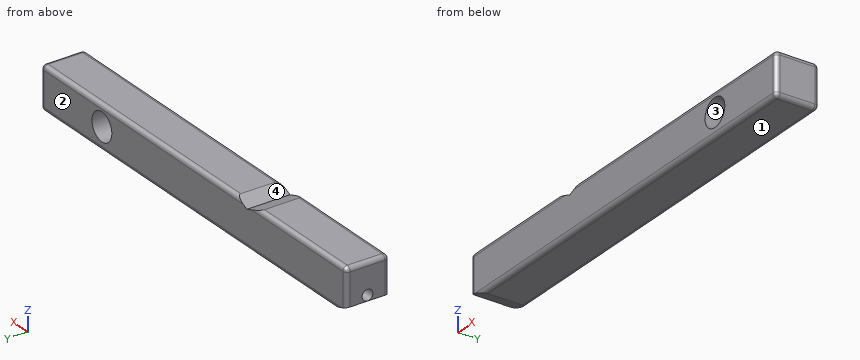
```python
from build123d import *

# Parameters (mm, degrees)
F0_R     = 3.25
F1_DEPTH = 10
F2_R     = 1.25
F3_DEPTH = 25
F4_R     = 1
F5_R     = 1


with BuildPart() as f1:
    # F0 (on Front) → F1 (new body)
    with BuildSketch(Plane.XZ):
        Polygon((-40.604423, 16.252205), (-36.365006, 14.785099), (59.395577, 14.785099), (59.395577, 24.785099), (-4.71925, 24.785099), (-8.140423, 23.253271), (-12.521202, 24.785099), (-40.604423, 24.785099), align=None)
        with Locations((39.395577, 20.006654)):
            Circle(F0_R, mode=Mode.SUBTRACT)
    extrude(amount=F1_DEPTH)

    # F2 (on face) → F3 (cut)
    with BuildSketch(Plane(origin=(-40.604423, 0, 0), x_dir=(0, -1, 0), z_dir=(-1, 0, 0))):
        with Locations((5, 17.535099)):
            Circle(F2_R)
    extrude(amount=-F3_DEPTH, mode=Mode.SUBTRACT)

    # F4
    f4_edges = [f1.edges().sort_by_distance(p)[0] for p in [
        (-26.562812, -10, 24.785099),
        (27.338164, -10, 24.785099),
        (27.338164, 0, 24.785099),
        (-26.562812, 0, 24.785099),
        (-40.604423, 0, 20.518652),
        (-40.604423, -5, 24.785099),
        (-40.604423, -10, 20.518652),
    ]]
    fillet(f4_edges, radius=F4_R)

    # F5
    f5_edges = [f1.edges().sort_by_distance(p)[0] for p in [
        (11.515286, -10, 14.785099),
        (11.515286, 0, 14.785099),
        (59.395577, -5, 24.785099),
        (59.395577, -0.292893, 24.492206),
        (59.395577, -9.707107, 24.492206),
        (59.395577, 0, 19.285099),
        (59.395577, -10, 19.285099),
        (59.395577, -5, 14.785099),
    ]]
    fillet(f5_edges, radius=F5_R)


solid = f1.part
```
Can you work these out from the model? Positions are in its coordinate system, mm. Face numbers are marked on the shaded views. Coordinates: 2 decimals unless noted, no trailing zeros. Loops run counter-clockwise (first coordinate to the right, second up) from the corner with the lowest first, then second, coordinate; pieces in that order, holes last. Notation, with made-up numbers: (-13, 18) - (32, 18) arc R10 ccw to (32, 36) - close; hole circle Ø10 at (-22, 23.5). An arc over 180 degrees is marked (long way). Answer as CSV lines item,"result". Start each with the question number.
1) Suppose I cut it at A-A (z = 22.25). Please give me the cut outline in (x, y), plus the area to 3 significant figures.
2) Suppose I cut it at C-C (x = -19). Please give me the cut outline in (y, z), plus the area to 3 significant figures.
3) Suppose I cut it at B-B (y = -5). Please give me the cut outline in (x, z) (3 decimals), plus the area to 3 significant figures.
4) Thinking about a two-plate mould opening in Z: for the marked faces 1, 2, 3 and 4, which applies, pulls with the +Z half, pulls with the -Z half, needs draft (parallel to the pull), parting line crosses it, or undercut?
5) For pin 1 (1.5 mm diameter, centred on y = -5, z = 17.54, fed in from -X), with a flat end and sliding along its axis, tell me the tip position at first contact or that it passes through.
6) I need wall thicknesses on line 1 (Z direction, x = -28.25, y = -5); line 2 (X direction, y = -8.25, z = 17.5); line 3 (X direction, y = -5, z = 22). Which ranges of each line are inside material? Lowest first, please. Write a range as from..to.
Check result:
1,outline,"(-40.6, -9) arc R1 ccw to (-39.6, -10) - (37.04, -10) - (37.04, 0) - (-39.6, 0) arc R1 ccw to (-40.6, -1) - close; (41.75, -10) - (58.4, -10) arc R1 ccw to (59.4, -9) - (59.4, -1) arc R1 ccw to (58.4, 0) - (41.75, 0) - close"
1,area,"952 mm²"
2,outline,"(-10, 15.79) arc R1 ccw to (-9, 14.79) - (-1, 14.79) arc R1 ccw to (0, 15.79) - (0, 23.79) arc R1 ccw to (-1, 24.79) - (-9, 24.79) arc R1 ccw to (-10, 23.79) - close; hole circle Ø2.5 at (-5, 17.54)"
2,area,"94.2 mm²"
3,outline,"(-40.604, 16.252) - (-36.365, 14.785) - (58.396, 14.785) arc R1 ccw to (59.396, 15.785) - (59.396, 23.785) arc R1 ccw to (58.396, 24.785) - (-4.719, 24.785) - (-8.14, 23.253) - (-12.521, 24.785) - (-39.604, 24.785) arc R1 ccw to (-40.604, 23.785) - (-40.604, 18.785) - (-15.604, 18.785) - (-15.604, 16.285) - (-40.604, 16.285) - close; hole circle Ø6.5 at (39.396, 20.007)"
3,area,"895 mm²"
4,face 1,"pulls with the -Z half"
4,face 2,"needs draft"
4,face 3,"undercut"
4,face 4,"pulls with the +Z half"
5,pin 1,"stops at x = -15.6"
6,line 1,"z = 14.79..16.29, 18.79..24.79"
6,line 2,"x = -40.6..37.33, 41.46..59.4"
6,line 3,"x = -40.6..36.83, 41.96..59.4"
